from build123d import *

# Parameters (mm, degrees)
SKETCH_1_W               = 3.183433307
SKETCH_1_H               = 0.999998
SKETCH_2_W               = 12.476289143
SKETCH_2_H               = 38.015688009
EXTRUDE_1_DEPTH          = 24.99995
SKETCH_3_W               = 12.476289143
SKETCH_3_H               = 24.99995
EXTRUDE_2_DEPTH          = 3.784228391
SKETCH_4_W               = 41.7999164
SKETCH_4_H               = 24.99995
EXTRUDE_3_DEPTH          = 51.023583857
SKETCH_6_W               = 21.499957
SKETCH_6_H               = 32.7999344
EXTRUDE_5_DEPTH          = 7.999984
SKETCH_7_W               = 11.999976
SKETCH_7_H               = 2.999994
CUT_EXTRUDE_1_DEPTH      = 8.999982
CUT_EXTRUDE_2_REACH      = 76.808
SKETCH_9_W               = 11.999976
SKETCH_9_H               = 2.999994
SKETCH_10_W              = 6.366689606
SKETCH_10_H              = 21.646744661
EXTRUDE_6_DEPTH          = 12.999974
SKETCH_11_W              = 11.999976
SKETCH_11_H              = 2.999994
CUT_EXTRUDE_3_DEPTH      = 11.999976
SKETCH_12_W              = 11.999976
SKETCH_12_H              = 2.999994
CUT_EXTRUDE_4_DEPTH      = 21.999956
SKETCH_13_W              = 11.999976
SKETCH_13_H              = 2.999994
CUT_EXTRUDE_5_DEPTH      = 11.999976
SKETCH_14_W              = 8.66186009
SKETCH_14_H              = 19.361804907
EXTRUDE_7_DEPTH          = 11.999976
SKETCH_15_W              = 3.82824354
SKETCH_15_H              = 0.999998
SKETCH_16_W              = 3.82824354
SKETCH_16_H              = 6
SKETCH_17_W              = 3.183433307
SKETCH_17_H              = 5.3
HOLE_WIZARD_M3_5_4_D     = 3.999992
HOLE_WIZARD_M3_5_4_DEPTH = 21.999956
HOLE_WIZARD_1_D          = 2.675202715
HOLE_WIZARD_1_DEPTH      = 21.499957
HOLE_WIZARD_M3_5_5_D     = 3.999992
HOLE_WIZARD_M3_5_5_DEPTH = 34.99993


with BuildPart() as part:
    # 草图1 → 旋转1 (revolve)
    with BuildSketch(Plane(origin=(0, 0, 6.967661698), x_dir=(-1, 0, 0), z_dir=(0, 0, -1)), mode=Mode.PRIVATE) as revolve_1_sk:
        with Locations((-10.88457249, 25.499949)):
            Rectangle(SKETCH_1_W, SKETCH_1_H)
    revolve(revolve_1_sk.sketch.rotate(Axis((9.292855836, 24.99995, 6.967661698), (0, 1, 0)), 270), axis=Axis((9.292855836, 24.99995, 6.967661698), (0, 1, 0)))

    # 草图2 → 凸台-拉伸1 (add)
    with BuildSketch(Plane(origin=(0, 24.99995, 0), x_dir=(1, 0, 0), z_dir=(0, 1, 0))):
        with Locations((6.238144572, -22.792072395)):
            Rectangle(SKETCH_2_W, SKETCH_2_H)
    extrude(amount=-EXTRUDE_1_DEPTH)

    # 草图3 → 凸台-拉伸2 (add)
    with BuildSketch(Plane(origin=(0, 0, 3.784228391), x_dir=(-1, 0, 0), z_dir=(0, 0, -1))):
        with Locations((-6.238144572, 12.499975)):
            Rectangle(SKETCH_3_W, SKETCH_3_H)
    extrude(amount=EXTRUDE_2_DEPTH)

    # 草图4 → 凸台-拉伸3 (add)
    with BuildSketch(Plane(origin=(12.476289143, 0, 0), x_dir=(0, 0, -1), z_dir=(1, 0, 0))):
        with Locations((-20.8999582, 12.499975)):
            Rectangle(SKETCH_4_W, SKETCH_4_H)
    extrude(amount=EXTRUDE_3_DEPTH)

    # 草图6 → 凸台-拉伸5 (add)
    with BuildSketch(Plane.XZ):
        with Locations((10.7499785, 16.3999672)):
            Rectangle(SKETCH_6_W, SKETCH_6_H)
    extrude(amount=EXTRUDE_5_DEPTH)

    # 草图7 → 切除-拉伸1 (cut)
    with BuildSketch(Plane.XY.offset(41.7999164)):
        with Locations((5.999988, 1.499997)):
            Rectangle(SKETCH_7_W, SKETCH_7_H)
    extrude(amount=-CUT_EXTRUDE_1_DEPTH, mode=Mode.SUBTRACT)

    # 草图9 → 切除-拉伸2 (cut, up to next)
    with BuildSketch(Plane(origin=(0, 0, 29.7999404), x_dir=(-1, 0, 0), z_dir=(0, 0, -1)), mode=Mode.PRIVATE) as cut_extrude_2_sk1:
        with Locations((-5.999988, 1.499997)):
            Rectangle(SKETCH_9_W, SKETCH_9_H)
    cut_extrude_2_tool1 = extrude(cut_extrude_2_sk1.sketch, amount=-CUT_EXTRUDE_2_REACH, mode=Mode.PRIVATE) & part.part
    add(cut_extrude_2_tool1.solids().sort_by_distance((5.999988, 1.499997, 29.79994))[0], mode=Mode.SUBTRACT)

    # 草图10 → 凸台-拉伸6 (add)
    with BuildSketch(Plane.XZ):
        with Locations((58.681033534, 23.637634731)):
            Rectangle(SKETCH_10_W, SKETCH_10_H)
    extrude(amount=EXTRUDE_6_DEPTH)

    # 草图11 → 切除-拉伸3 (cut)
    with BuildSketch(Plane.XY.offset(41.7999164)):
        with Locations((5.999988, 23.499953)):
            Rectangle(SKETCH_11_W, SKETCH_11_H)
    extrude(amount=-CUT_EXTRUDE_3_DEPTH, mode=Mode.SUBTRACT)

    # 草图12 → 切除-拉伸4 (cut)
    with BuildSketch(Plane(origin=(63.499873, 0, 0), x_dir=(0, 0, -1), z_dir=(1, 0, 0))):
        with Locations((-5.999988, 23.499953)):
            Rectangle(SKETCH_12_W, SKETCH_12_H)
    extrude(amount=-CUT_EXTRUDE_4_DEPTH, mode=Mode.SUBTRACT)

    # 草图13 → 切除-拉伸5 (cut)
    with BuildSketch(Plane(origin=(63.499873, 0, 0), x_dir=(0, 0, -1), z_dir=(1, 0, 0))):
        with Locations((-5.999988, 1.499997)):
            Rectangle(SKETCH_13_W, SKETCH_13_H)
    extrude(amount=-CUT_EXTRUDE_5_DEPTH, mode=Mode.SUBTRACT)

    # 草图14 → 凸台-拉伸7 (add)
    with BuildSketch(Plane.XZ):
        with Locations((50.029008896, 22.492211894)):
            Rectangle(SKETCH_14_W, SKETCH_14_H)
    extrude(amount=EXTRUDE_7_DEPTH)

    # 草图15 → 旋转2 (revolve)
    with BuildSketch(Plane(origin=(0, 0, 34.32537348), x_dir=(-1, 0, 0), z_dir=(0, 0, -1)), mode=Mode.PRIVATE) as revolve_2_sk:
        with Locations((-35.382002405, 25.499949)):
            Rectangle(SKETCH_15_W, SKETCH_15_H)
    revolve(revolve_2_sk.sketch.rotate(Axis((33.467880635, 24.99995, 34.32537348), (0, 1, 0)), 270), axis=Axis((33.467880635, 24.99995, 34.32537348), (0, 1, 0)))

    # 草图16 → 旋转3 (revolve)
    with BuildSketch(Plane(origin=(0, 0, 23.254177941), x_dir=(-1, 0, 0), z_dir=(0, 0, -1)), mode=Mode.PRIVATE) as revolve_3_sk:
        with Locations((-35.382002405, 27.99995)):
            Rectangle(SKETCH_16_W, SKETCH_16_H)
    revolve(revolve_3_sk.sketch.rotate(Axis((33.467880635, 24.99995, 23.254177941), (0, 1, 0)), 270), axis=Axis((33.467880635, 24.99995, 23.254177941), (0, 1, 0)))

    # 草图17 → 旋转4 (revolve)
    with BuildSketch(Plane(origin=(0, 0, 6.967661698), x_dir=(-1, 0, 0), z_dir=(0, 0, -1)), mode=Mode.PRIVATE) as revolve_4_sk:
        with Locations((-27.552434059, 27.64995)):
            Rectangle(SKETCH_17_W, SKETCH_17_H)
    revolve(revolve_4_sk.sketch.rotate(Axis((25.960717405, 24.99995, 6.967661698), (0, 1, 0)), 270), axis=Axis((25.960717405, 24.99995, 6.967661698), (0, 1, 0)))

    # M3.5 间隙孔4
    with Locations(Plane(origin=(0, 24.99995, 0), x_dir=(1, 0, 0), z_dir=(0, 1, 0))):
        with Locations((58.499883, -35.7999284)):
            Hole(HOLE_WIZARD_M3_5_4_D / 2, depth=HOLE_WIZARD_M3_5_4_DEPTH)

    # 孔1
    with Locations(Plane(origin=(21.499957, 0, 0), x_dir=(0, 0, -1), z_dir=(1, 0, 0))):
        with Locations((-16.500963355, -3.875126559), (-21.645583961, -3.875126559), (-26.069957682, -3.875126559), (-30.391438991, -3.875126559), (-11.870804809, -3.875126559), (-7.858000737, -3.875126559), (-3.227842192, -3.875126559)):
            Hole(HOLE_WIZARD_1_D / 2, depth=HOLE_WIZARD_1_DEPTH)

    # M3.5 间隙孔5
    with Locations(Plane(origin=(0, 21.999956, 0), x_dir=(1, 0, 0), z_dir=(0, 1, 0))):
        with Locations((58.499883, -5.999988), (4.99999, -35.7999284)):
            Hole(HOLE_WIZARD_M3_5_5_D / 2, depth=HOLE_WIZARD_M3_5_5_DEPTH)


solid = part.part
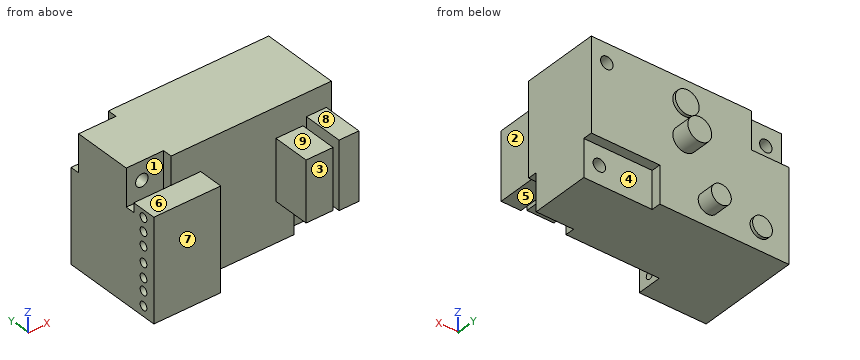
For this review, take the finished solid that the model builds, in its own axes (mm). Face numbers are marked on the shaded views. A direction names the side the tool comes from. Round coordinates to 2 decimals unless told otherwise and drop trailing zeros. Order: outer loops, then holes, each group sorted by start corner. A loop starts at its lowest first (then second) coordinate and runs counter-clockwise, first axis right, second up. Notation, with made-up numbers: M 14.25,84 L 53.25,84 A18 ccw 53.25,91 Z; hole C -36,72 d6. An arc over 180 degrees is marked long. Use a Markdown table: item, result. Add a question column.
Item 1: Add section C-C, the plane x = 8. Give the boundary of the cut face in (y, z), then the cut area to 3 significant figures.
Item 2: Add section A-A, the plane y = 24. Give the boundary of the cut face in (x, z), then the cut area to 3 significant figures.
Item 3: Mouldability with a two-part tool opening along Y and no side actions: class the marked faces 1, 2, 3 and 4 as released by +Y, released by -Y, zero draft, split by the parting line, or undercut.
Item 4: Add section D-D, the plane x = 27.5. Give the boundary of the cut face in (y, z).
Item 5: Tool access review of the marked faces 5, 6, 7, 8 and 9: name each direction out of +Z, -Z, +X, -X, +Y, -Y from which nothing blocks a thin tool from reaching the whole face with its end or side.
Item 6: Add section B-B, the plane z = 3. Give the boundary of the cut face in (x, y), then the cut area to 3 significant figures.
Item 7: To check wall thickness, follow line 1 along X through (y, z) = (-2, 18); line 2 along Z through (x, y) = (5, 10); line 3 along Y through (x, z) = (4.5, 26). State the ranges of each line that lie inside material, in increasing order.
Item 8: Insertion check: pin 1 (6.5 mm diameter, centred on x = 6, z = 18.5, fed in from -Y); pin 2 (9.5 mm diameter, centred on x = 58.5, z = 5, fed in from -Y); pin 3 (12 mm diameter, centred on x = 15, y = -3.5, fed in from -Z); pin 4 (3 mm diameter, centred on x = 58.5, z = 35.5, fed in from +Y). Each pin has a flat end and moves straight along its axis. Give the tip position at first contact, or say it passes through.
Geometry results:
| question | item | result |
|---|---|---|
| 1 | outline | M -8,0 L 25,0 L 25,4.06 L 26,4.06 L 26,9.88 L 25,9.88 L 25,29.8 L 22,29.8 L 22,41.8 L 3,41.8 L 3,29.8 L 0,29.8 L 0,32.8 L -8,32.8 Z; hole C -3.88,3.23 d2.68; hole C -3.88,7.86 d2.68; hole C -3.88,11.87 d2.68; hole C -3.88,16.5 d2.68; hole C -3.88,21.65 d2.68; hole C -3.88,26.07 d2.68; hole C -3.88,30.39 d2.68 |
| 1 | area | 1,200 mm² |
| 2 | outline | M 0,0 L 41.5,0 L 41.5,12 L 63.5,12 L 63.5,41.8 L 12,41.8 L 12,29.8 L 0,29.8 Z; hole C 58.5,35.8 d4 |
| 2 | area | 2,230 mm² |
| 3 | face 1 | undercut |
| 3 | face 2 | zero draft |
| 3 | face 3 | released by -Y |
| 3 | face 4 | released by +Y |
| 4 | outline | M 0,0 L 25,0 L 25,4.18 L 30.3,4.18 L 30.3,9.75 L 25,9.75 L 25,41.8 L 0,41.8 Z |
| 5 | face 5 | -Z, +X, -Y |
| 5 | face 6 | +Z, -X, -Y |
| 5 | face 7 | +Z, -Z, -X, -Y |
| 5 | face 8 | +Z, +X, -X, -Y |
| 5 | face 9 | +Z, -Y |
| 6 | outline | M 0,-8 L 21.5,-8 L 21.5,-5.19 L 0,-5.19 Z; M 0,-2.56 L 21.5,-2.56 L 21.5,0 L 51.5,0 L 51.5,3 L 63.5,3 L 63.5,22 L 41.5,22 L 41.5,25 L 0,25 Z |
| 6 | area | 1,600 mm² |
| 7 | line 1 | x = 0 to 21.5, 45.7 to 54.36, 55.5 to 61.86 |
| 7 | line 2 | z = 0 to 33.8, 37.8 to 41.8 |
| 7 | line 3 | y = -8 to -5.21, -2.54 to 25 |
| 8 | pin 1 | stops at y = -8 |
| 8 | pin 2 | stops at y = 3 |
| 8 | pin 3 | stops at z = 0 |
| 8 | pin 4 | stops at y = 3 |
